from build123d import *

# Parameters (mm, degrees)
BOSS_EXTRUDE1_DEPTH             = 3.175
F_6_CLEARANCE_HOLE1_AT_2_COUNT  = 2
F_6_CLEARANCE_HOLE1_AT_2_PITCH  = 202.184
F_6_CLEARANCE_HOLE1_AT_3_COUNT  = 2
F_6_CLEARANCE_HOLE1_AT_3_PITCH  = 245.533205315
F_6_CLEARANCE_HOLE1_AT_4_COUNT  = 2
F_6_CLEARANCE_HOLE1_AT_4_PITCH  = 294.732330958
F_6_CLEARANCE_HOLE1_AT_5_COUNT  = 2
F_6_CLEARANCE_HOLE1_AT_5_PITCH  = 209.296
F_6_CLEARANCE_HOLE1_AT_6_COUNT  = 2
F_6_CLEARANCE_HOLE1_AT_6_PITCH  = 172.811757411
F_6_CLEARANCE_HOLE1_AT_7_COUNT  = 2
F_6_CLEARANCE_HOLE1_AT_7_PITCH  = 57.300187604
F_6_CLEARANCE_HOLE1_AT_8_COUNT  = 2
F_6_CLEARANCE_HOLE1_AT_8_PITCH  = 291.003755082
F_6_CLEARANCE_HOLE1_AT_9_COUNT  = 2
F_6_CLEARANCE_HOLE1_AT_9_PITCH  = 232.431512666
F_6_CLEARANCE_HOLE1_AT_10_COUNT = 2
F_6_CLEARANCE_HOLE1_AT_10_PITCH = 101.092
SKETCH23_R                      = 24.765
CUT_EXTRUDE10_DEPTH             = 191.76187976
SKETCH24_W                      = 59.69
SKETCH24_H                      = 45.212
CUT_EXTRUDE11_DEPTH             = 191.76187976
FILLET2_R                       = 4.699
CHAMFER1_SIZE                   = 1.905
M3_CLEARANCE_HOLE3_AT_2_COUNT   = 2
M3_CLEARANCE_HOLE3_AT_2_PITCH   = 49.391408666
M3_CLEARANCE_HOLE3_AT_3_COUNT   = 2
M3_CLEARANCE_HOLE3_AT_3_PITCH   = 69.85
M3_CLEARANCE_HOLE3_AT_4_COUNT   = 2
M3_CLEARANCE_HOLE3_AT_4_PITCH   = 49.391408666
M3_CLEARANCE_HOLE1_D            = 3.6
M3_CLEARANCE_HOLE1_CSINK_D      = 5.7
M3_CLEARANCE_HOLE1_CSINK_ANGLE  = 90
M3_CLEARANCE_HOLE2_AT_2_COUNT   = 2
M3_CLEARANCE_HOLE2_AT_2_PITCH   = 56.70042
M3_CLEARANCE_HOLE2_AT_3_COUNT   = 2
M3_CLEARANCE_HOLE2_AT_3_PITCH   = 102.00589147
M3_CLEARANCE_HOLE2_AT_4_COUNT   = 2
M3_CLEARANCE_HOLE2_AT_4_PITCH   = 109.267844742
M3_CLEARANCE_HOLE2_AT_5_COUNT   = 2
M3_CLEARANCE_HOLE2_AT_5_PITCH   = 65.600653918
M3_CLEARANCE_HOLE2_AT_6_COUNT   = 2
M3_CLEARANCE_HOLE2_AT_6_PITCH   = 76.404880698
M3_CLEARANCE_HOLE2_AT_7_COUNT   = 2
M3_CLEARANCE_HOLE2_AT_7_PITCH   = 27.404059918
M3_CLEARANCE_HOLE2_AT_8_COUNT   = 2
M3_CLEARANCE_HOLE2_AT_8_PITCH   = 55.968061912
SKETCH35_W                      = 13.335
SKETCH35_H                      = 28.575
CUT_EXTRUDE12_DEPTH             = 191.76187976
FILLET1_R                       = 1.5875
F_8_0MM_DOWEL_HOLE1_D           = 8
M3_CLEARANCE_HOLE4_AT_2_COUNT   = 2
M3_CLEARANCE_HOLE4_AT_2_PITCH   = 78.105
M3_CLEARANCE_HOLE4_AT_3_COUNT   = 2
M3_CLEARANCE_HOLE4_AT_3_PITCH   = 97.157075141
M3_CLEARANCE_HOLE4_AT_4_COUNT   = 2
M3_CLEARANCE_HOLE4_AT_4_PITCH   = 57.785
SKETCH42_OUTSIDE_W              = 382.23
SKETCH42_OUTSIDE_H              = 308.826
SKETCH42_OUTSIDE_W_2            = 133.096408578
SKETCH42_OUTSIDE_H_2            = 80.832743403
CUT_EXTRUDE13_DEPTH             = 191.76187976
FILLET3_R                       = 6.35


with BuildPart() as part:
    # Sketch1 → Boss-Extrude1 (new body)
    with BuildSketch(Plane.XY):
        with BuildLine():
            Line((-151.96693, 98.7552), (-151.96693, -98.7552))
            ThreePointArc((-151.96693, -98.7552), (-147.131262957, -110.429532957), (-135.45693, -115.2652))
            Line((-135.45693, -115.2652), (135.45693, -115.2652))
            ThreePointArc((135.45693, -115.2652), (147.131262957, -110.429532957), (151.96693, -98.7552))
            Line((151.96693, -98.7552), (151.96693, 98.7552))
            ThreePointArc((151.96693, 98.7552), (147.131262957, 110.429532957), (135.45693, 115.2652))
            Line((135.45693, 115.2652), (-135.45693, 115.2652))
            ThreePointArc((-135.45693, 115.2652), (-147.131262957, 110.429532957), (-151.96693, 98.7552))
        make_face()
    extrude(amount=-BOSS_EXTRUDE1_DEPTH)

    # Sketch3 → #6 Clearance Hole1 (revolve, cut)
    with BuildSketch(Plane(origin=(101.092, 104.648, 0), x_dir=(0, -1, 0), z_dir=(1, 0, 0))):
        Polygon((0, 0), (0, 3.175), (3.3655, 3.175), (2.15265, 2.157298012), (2.15265, 0), align=None)
    f_6_clearance_hole1 = revolve(axis=Axis((101.092, 104.648, 6.35), (0, 0, -1)), mode=Mode.SUBTRACT)

    # #6 Clearance Hole1 at 2: #6 Clearance Hole1 ×2
    with Locations(*[(-i * F_6_CLEARANCE_HOLE1_AT_2_PITCH, 0, 0) for i in range(1, F_6_CLEARANCE_HOLE1_AT_2_COUNT)]):
        add(f_6_clearance_hole1, mode=Mode.SUBTRACT)

    # #6 Clearance Hole1 at 3: #6 Clearance Hole1 ×2
    with Locations(*[Vector(-0.9858574105677721, -0.1675862942743448, 0) * (i * F_6_CLEARANCE_HOLE1_AT_3_PITCH) for i in range(1, F_6_CLEARANCE_HOLE1_AT_3_COUNT)]):
        add(f_6_clearance_hole1, mode=Mode.SUBTRACT)

    # #6 Clearance Hole1 at 4: #6 Clearance Hole1 ×2
    with Locations(*[Vector(-0.8212900471859665, -0.5705108749123656, 0) * (i * F_6_CLEARANCE_HOLE1_AT_4_PITCH) for i in range(1, F_6_CLEARANCE_HOLE1_AT_4_COUNT)]):
        add(f_6_clearance_hole1, mode=Mode.SUBTRACT)

    # #6 Clearance Hole1 at 5: #6 Clearance Hole1 ×2
    with Locations(*[(0, -i * F_6_CLEARANCE_HOLE1_AT_5_PITCH, 0) for i in range(1, F_6_CLEARANCE_HOLE1_AT_5_COUNT)]):
        add(f_6_clearance_hole1, mode=Mode.SUBTRACT)

    # #6 Clearance Hole1 at 6: #6 Clearance Hole1 ×2
    with Locations(*[Vector(0.23075241289949347, -0.9730124993755537, 0) * (i * F_6_CLEARANCE_HOLE1_AT_6_PITCH) for i in range(1, F_6_CLEARANCE_HOLE1_AT_6_COUNT)]):
        add(f_6_clearance_hole1, mode=Mode.SUBTRACT)

    # #6 Clearance Hole1 at 7: #6 Clearance Hole1 ×2
    with Locations(*[Vector(0.6959266918172804, -0.7181128320927402, 0) * (i * F_6_CLEARANCE_HOLE1_AT_7_PITCH) for i in range(1, F_6_CLEARANCE_HOLE1_AT_7_COUNT)]):
        add(f_6_clearance_hole1, mode=Mode.SUBTRACT)

    # #6 Clearance Hole1 at 8: #6 Clearance Hole1 ×2
    with Locations(*[Vector(-0.6947814125038304, -0.719220959677332, 0) * (i * F_6_CLEARANCE_HOLE1_AT_8_PITCH) for i in range(1, F_6_CLEARANCE_HOLE1_AT_8_COUNT)]):
        add(f_6_clearance_hole1, mode=Mode.SUBTRACT)

    # #6 Clearance Hole1 at 9: #6 Clearance Hole1 ×2
    with Locations(*[Vector(-0.4349324187613887, -0.9004630981391565, 0) * (i * F_6_CLEARANCE_HOLE1_AT_9_PITCH) for i in range(1, F_6_CLEARANCE_HOLE1_AT_9_COUNT)]):
        add(f_6_clearance_hole1, mode=Mode.SUBTRACT)

    # #6 Clearance Hole1 at 10: #6 Clearance Hole1 ×2
    with Locations(*[(-i * F_6_CLEARANCE_HOLE1_AT_10_PITCH, 0, 0) for i in range(1, F_6_CLEARANCE_HOLE1_AT_10_COUNT)]):
        add(f_6_clearance_hole1, mode=Mode.SUBTRACT)

    # Sketch23 → Cut-Extrude10 (cut, through all)
    with BuildSketch(Plane.XY):
        with Locations((104.26573, 42.164)):
            Circle(SKETCH23_R)
    extrude(amount=-CUT_EXTRUDE10_DEPTH, mode=Mode.SUBTRACT)

    # Sketch24 → Cut-Extrude11 (cut, through all)
    with BuildSketch(Plane.XY):
        with Locations((-63.06693, 16.31442)):
            Rectangle(SKETCH24_W, SKETCH24_H)
    extrude(amount=-CUT_EXTRUDE11_DEPTH, mode=Mode.SUBTRACT)

    # Fillet2
    fillet2_edges = [part.edges().sort_by_distance(p)[0] for p in [
        (-92.91193, -6.29158, -1.5875),
        (-92.91193, 38.92042, -1.5875),
        (-33.22193, 38.92042, -1.5875),
        (-33.22193, -6.29158, -1.5875),
    ]]
    fillet(fillet2_edges, radius=FILLET2_R)

    # Chamfer1
    chamfer1_edges = [part.edges().sort_by_distance(p)[0] for p in [
        (-33.22193, 16.31442, -3.175),
        (-63.06693, -6.29158, -3.175),
        (-92.91193, 16.31442, -3.175),
        (-63.06693, 38.92042, -3.175),
        (-34.598235235, -4.915274765, -3.175),
        (-91.535624765, -4.915274765, -3.175),
        (-91.535624765, 37.544114765, -3.175),
        (-34.598235235, 37.544114765, -3.175),
    ]]
    chamfer(chamfer1_edges, length=CHAMFER1_SIZE)

    # Sketch30 → M3 Clearance Hole3 (revolve, cut)
    with BuildSketch(Plane(origin=(79.570025667, 66.859704333, 0), x_dir=(0, -1, 0), z_dir=(1, 0, 0))):
        Polygon((0, 0), (0, 3.175), (2.85, 3.175), (1.8, 2.125), (1.8, 0), align=None)
    m3_clearance_hole3 = revolve(axis=Axis((79.570025667, 66.859704333, 6.35), (0, 0, -1)), mode=Mode.SUBTRACT)

    # M3 Clearance Hole3 at 2: M3 Clearance Hole3 ×2
    with Locations(*[(i * M3_CLEARANCE_HOLE3_AT_2_PITCH, 0, 0) for i in range(1, M3_CLEARANCE_HOLE3_AT_2_COUNT)]):
        add(m3_clearance_hole3, mode=Mode.SUBTRACT)

    # M3 Clearance Hole3 at 3: M3 Clearance Hole3 ×2
    with Locations(*[Vector(0.7071067811865477, -0.7071067811865475, 0) * (i * M3_CLEARANCE_HOLE3_AT_3_PITCH) for i in range(1, M3_CLEARANCE_HOLE3_AT_3_COUNT)]):
        add(m3_clearance_hole3, mode=Mode.SUBTRACT)

    # M3 Clearance Hole3 at 4: M3 Clearance Hole3 ×2
    with Locations(*[(0, -i * M3_CLEARANCE_HOLE3_AT_4_PITCH, 0) for i in range(1, M3_CLEARANCE_HOLE3_AT_4_COUNT)]):
        add(m3_clearance_hole3, mode=Mode.SUBTRACT)

    # M3 Clearance Hole1 (through all)
    with Locations(Plane(origin=(0, 0, -3.175), x_dir=(-1, 0, 0), z_dir=(0, 0, -1))):
        with Locations((17.67693, -38.5952), (117.67693, -38.5952), (117.67693, -88.5952), (17.67693, -88.5952)):
            CounterSinkHole(M3_CLEARANCE_HOLE1_D / 2, M3_CLEARANCE_HOLE1_CSINK_D / 2, counter_sink_angle=M3_CLEARANCE_HOLE1_CSINK_ANGLE)

    # Sketch34 → M3 Clearance Hole2 (revolve, cut)
    with BuildSketch(Plane(origin=(25.25193, -75.5297, 0), x_dir=(0, -1, 0), z_dir=(1, 0, 0))):
        Polygon((0, 0), (0, 3.175), (2.85, 3.175), (1.8, 2.125), (1.8, 0), align=None)
    m3_clearance_hole2 = revolve(axis=Axis((25.25193, -75.5297, 6.35), (0, 0, -1)), mode=Mode.SUBTRACT)

    # M3 Clearance Hole2 at 2: M3 Clearance Hole2 ×2
    with Locations(*[(i * M3_CLEARANCE_HOLE2_AT_2_PITCH, 0, 0) for i in range(1, M3_CLEARANCE_HOLE2_AT_2_COUNT)]):
        add(m3_clearance_hole2, mode=Mode.SUBTRACT)

    # M3 Clearance Hole2 at 3: M3 Clearance Hole2 ×2
    with Locations(*[Vector(0.9983315525499471, -0.05774176290357108, 0) * (i * M3_CLEARANCE_HOLE2_AT_3_PITCH) for i in range(1, M3_CLEARANCE_HOLE2_AT_3_COUNT)]):
        add(m3_clearance_hole2, mode=Mode.SUBTRACT)

    # M3 Clearance Hole2 at 4: M3 Clearance Hole2 ×2
    with Locations(*[Vector(0.9319823250907686, 0.36250371821321364, 0) * (i * M3_CLEARANCE_HOLE2_AT_4_PITCH) for i in range(1, M3_CLEARANCE_HOLE2_AT_4_COUNT)]):
        add(m3_clearance_hole2, mode=Mode.SUBTRACT)

    # M3 Clearance Hole2 at 5: M3 Clearance Hole2 ×2
    with Locations(*[Vector(0.9959611085814934, -0.089785690358334, 0) * (i * M3_CLEARANCE_HOLE2_AT_5_PITCH) for i in range(1, M3_CLEARANCE_HOLE2_AT_5_COUNT)]):
        add(m3_clearance_hole2, mode=Mode.SUBTRACT)

    # M3 Clearance Hole2 at 6: M3 Clearance Hole2 ×2
    with Locations(*[Vector(0.8551246910281444, 0.5184223787550272, 0) * (i * M3_CLEARANCE_HOLE2_AT_6_PITCH) for i in range(1, M3_CLEARANCE_HOLE2_AT_6_COUNT)]):
        add(m3_clearance_hole2, mode=Mode.SUBTRACT)

    # M3 Clearance Hole2 at 7: M3 Clearance Hole2 ×2
    with Locations(*[Vector(0.2682084341495708, 0.9633609063331537, 0) * (i * M3_CLEARANCE_HOLE2_AT_7_PITCH) for i in range(1, M3_CLEARANCE_HOLE2_AT_7_COUNT)]):
        add(m3_clearance_hole2, mode=Mode.SUBTRACT)

    # M3 Clearance Hole2 at 8: M3 Clearance Hole2 ×2
    with Locations(*[Vector(0.8817603882311722, 0.47169759141468215, 0) * (i * M3_CLEARANCE_HOLE2_AT_8_PITCH) for i in range(1, M3_CLEARANCE_HOLE2_AT_8_COUNT)]):
        add(m3_clearance_hole2, mode=Mode.SUBTRACT)

    # Sketch35 → Cut-Extrude12 (cut, through all)
    with BuildSketch(Plane.XY):
        with Locations((-126.56693, 16.8402)):
            Rectangle(SKETCH35_W, SKETCH35_H)
    extrude(amount=-CUT_EXTRUDE12_DEPTH, mode=Mode.SUBTRACT)

    # Fillet1
    fillet1_edges = [part.edges().sort_by_distance(p)[0] for p in [
        (-133.23443, 2.5527, -1.5875),
        (-133.23443, 31.1277, -1.5875),
        (-119.89943, 31.1277, -1.5875),
        (-119.89943, 2.5527, -1.5875),
    ]]
    fillet(fillet1_edges, radius=FILLET1_R)

    # Ø8.0mm Dowel Hole1 (through all)
    with Locations(Plane(origin=(0, 0, -3.175), x_dir=(-1, 0, 0), z_dir=(0, 0, -1))):
        with Locations((12.26693, 3.61442), (12.26693, 29.01442)):
            Hole(F_8_0MM_DOWEL_HOLE1_D / 2)

    # Sketch39 → M3 Clearance Hole4 (revolve, cut)
    with BuildSketch(Plane(origin=(-105.23093, 45.65142, 0), x_dir=(0, -1, 0), z_dir=(1, 0, 0))):
        Polygon((0, 0), (0, 3.175), (2.85, 3.175), (1.7, 2.025), (1.7, 0), align=None)
    m3_clearance_hole4 = revolve(axis=Axis((-105.23093, 45.65142, 6.35), (0, 0, -1)), mode=Mode.SUBTRACT)

    # M3 Clearance Hole4 at 2: M3 Clearance Hole4 ×2
    with Locations(*[(i * M3_CLEARANCE_HOLE4_AT_2_PITCH, 0, 0) for i in range(1, M3_CLEARANCE_HOLE4_AT_2_COUNT)]):
        add(m3_clearance_hole4, mode=Mode.SUBTRACT)

    # M3 Clearance Hole4 at 3: M3 Clearance Hole4 ×2
    with Locations(*[Vector(0.8039043979705941, -0.5947585383359678, 0) * (i * M3_CLEARANCE_HOLE4_AT_3_PITCH) for i in range(1, M3_CLEARANCE_HOLE4_AT_3_COUNT)]):
        add(m3_clearance_hole4, mode=Mode.SUBTRACT)

    # M3 Clearance Hole4 at 4: M3 Clearance Hole4 ×2
    with Locations(*[(0, -i * M3_CLEARANCE_HOLE4_AT_4_PITCH, 0) for i in range(1, M3_CLEARANCE_HOLE4_AT_4_COUNT)]):
        add(m3_clearance_hole4, mode=Mode.SUBTRACT)

    # Sketch42 outside → Cut-Extrude13 (cut, through all)
    with BuildSketch(Plane(origin=(0, 0, -3.175), x_dir=(-1, 0, 0), z_dir=(0, 0, -1))):
        Rectangle(SKETCH42_OUTSIDE_W, SKETCH42_OUTSIDE_H)
        with Locations((85.418725711, 15.951898655)):
            Rectangle(SKETCH42_OUTSIDE_W_2, SKETCH42_OUTSIDE_H_2, mode=Mode.SUBTRACT)
    extrude(amount=-CUT_EXTRUDE13_DEPTH, mode=Mode.SUBTRACT)

    # Fillet3
    fillet3_edges = [part.edges().sort_by_distance(p)[0] for p in [
        (-18.870521422, 56.368270356, -1.5875),
        (-151.96693, 56.368270356, -1.5875),
        (-151.96693, -24.464473047, -1.5875),
        (-18.870521422, -24.464473047, -1.5875),
    ]]
    fillet(fillet3_edges, radius=FILLET3_R)


solid = part.part
Could you check a few things on this model? Use its own coordinates, in mm. A direction names the side the tool comes from. Coordinates: 2 decimals unless noted, no trailing zeros. Loops run counter-clockwise (first coordinate to the right, second up) from the corner with the lowest first, then second, coordinate; pieces in that order, holes last.
1. Imagine slicing it at C-C (z = -0.65). Give the number of separate pieces and of enclosed holes in the cut face, and give its area (3 significant figures).
2. I need wall thicknesses on L1, parallel to X at y = 18.5, z = -0.2; L2, parallel to X at y = 30, z = -1.2; L3, parallel to Y at x = -67, z = -2.9. Which ranges of each line are inside material? Lowest first, please.
3. We'd pull the mould along X, two halves only. Please class faces 1 (the face through (-34.11, -5.49, -2.02)), 2 (the face through (-101, 17, 0)), 3 (the face through (-20.78, 54.56, -1.57)): released by +X, released by -X, zero draft, split by the parting line, or undercut.
4. Imagine slicing it at D-D (x = -123.5). Please give me the cut outline in (y, z) (3 decimals), and give its area (3 significant figures).
5. For P1, Ø4, axis at x = -105.23, y = -12.13, coming from the -Z side; P2, Ø3, axis at x = -27.13, y = -12.13, coming from the -Z side; P3, Ø5.5, axis at x = -27.13, y = 45.65, coming from the +Z side, each with a flat end and sliding along its axis, tell me the tip position at first contact or that it passes through.
6. Imagine slicing it at A-A (y = 8.5). Please give me the cut outline in (x, z) (3 decimals).
7. Imagine slicing it at B-B (x = -41). Please give me the cut outline in (y, z) (3 decimals), and give its area (3 significant figures).
8. For faces 4 (the face through (-92.111, -5.406, -2.024)), 5 (the face through (-127, 2.553, -2)), 6 (the face through (-18.871, 15, -2)), which set-ups out of +Z, -Z, +X, -X, +Y, -Y let a thin tool reach every point of the face, with its end or its side?
Computed values:
1. separate pieces: 1
1. enclosed holes: 6
1. area: 7,630 mm2
2. L1: x = -151.97 to -133.23, -119.9 to -92.91, -33.22 to -18.87
2. L2: x = -151.97 to -133.17, -119.97 to -92.91, -33.22 to -18.87
2. L3: y = -24.46 to -7.92, 40.55 to 56.37
3. face 1: undercut
3. face 2: zero draft
3. face 3: released by +X
4. outline: (-24.464, -3.175) - (2.553, -3.175) - (2.553, 0) - (-24.464, 0) - close; (31.128, -3.175) - (56.368, -3.175) - (56.368, 0) - (31.128, 0) - close
4. area: 166 mm2
5. P1: stops at z = -2.33
5. P2: passes through
5. P3: stops at z = 0
6. outline: (-151.967, -3.175) - (-133.234, -3.175) - (-133.234, 0) - (-151.967, 0) - close; (-119.899, -3.175) - (-94.817, -3.175) - (-92.912, -1.27) - (-92.912, 0) - (-119.899, 0) - close; (-33.222, -1.27) - (-31.317, -3.175) - (-18.871, -3.175) - (-18.871, 0) - (-33.222, 0) - close
7. outline: (-24.464, -3.175) - (-8.197, -3.175) - (-6.292, -1.27) - (-6.292, 0) - (-24.464, 0) - close; (38.92, -1.27) - (40.825, -3.175) - (56.368, -3.175) - (56.368, 0) - (38.92, 0) - close
7. area: 109 mm2
8. face 4: -Z
8. face 5: +Z, -Z
8. face 6: +Z, -Z, +X, +Y, -Y
